Read the model definition and answer for the solid it produces. Units are mm, in the model's axes. Face numbers are marked on the shaded views. A direction names the side the tool comes from. Coordinates: 2 decimals unless noted, no trailing zeros. Write each loop counter-clockwise with the first axis right and the second up, starting at its lowest first coordinate (ties: lowest second). Pieces come first, ordered by that corner, then holes. Notation, with made-up numbers: (29.25, 33) -> (37.25, 33) arc R16 ccw to (37.25, 63) -> close; hole circle Ø10 at (-35, -17). An arc over 180 degrees is marked (long way). Write item = value, one per line. Start each with the question number.
1) Section B-B (z = 3) is taken. Determine the outline of the cut face in (x, y).
2) Find the intervals of material crossed by line 1 along X through (y, z) = (138, 6.75); line 2 along X through (y, z) = (12.5, 5), in increasing order. Write a range as from..to.
3) Section C-C (y = 113.5) is taken. Determine the outline of the cut face in (x, z).
4) Section D-D (y = 40.5) is taken. Determine the outline of the cut face in (x, z), plus the area to 3 significant figures.
5) A tool of negligible diameter and unlimited length cuts with its end or side. For the marked faces 1 and 2, from which of +Z, -Z, +X, -X, +Y, -Y can it reach the whole face along a straight path? Write none if from no direction.
6) Section A-A (x = -9.5) is taken. Determine the outline of the cut face in (y, z), plus the area to 3 significant figures.
7) Flat-ended cylindrical pins translate along their axes: pin 1 Ø1 at (y, z) = (78.5, 4.5) entering from +X; pin 2 Ø3.5 at (y, z) = (-0.5, 4) entering from -X; pin 3 Ø6 at (x, y) = (-15, 128) entering from -Z; pin 4 Ø2 at (y, z) = (-0.5, 2) entering from +X. Find the tip coordinate at first contact, or state that the pin passes through.
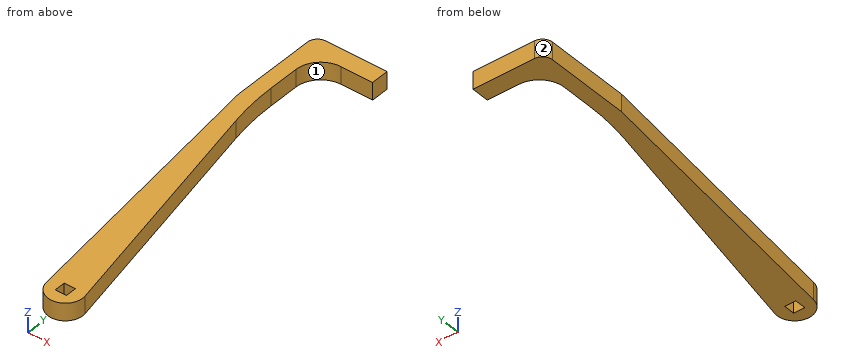
Autodesk Inventor part; units mm, degrees
ref_plane "YZ Plane" through (0, 0, 0) normal (1, 0, 0) x (0, 1, 0)
ref_plane "XZ Plane" through (0, 0, 0) normal (0, 1, 0) x (-1, 0, 0)
ref_plane "XY Plane" through (0, 0, 0) normal (0, 0, 1) x (1, 0, 0)
sketch "Эскиз1" plane through (0, 0, 0) normal (0, 0, 1) x (1, 0, 0)
  circle A0 centre (0.0899, -0.0505) radius 4
  line L0 (-20.8576, 111.2941) -> (-20.8576, 149.3795)
  line L1 (-20.8576, 149.3795) -> (-6.2988, 149.3795)
  line L2 (7.9099, 149.3795) -> (-6.2988, 149.3795)
  line L3 (-14.8576, 142.2545) -> (7.9099, 142.2545)
  line L4 (-14.8576, 142.2545) -> (7.9099, 142.2545)
  line L5 (-14.8576, 109.9334) -> (-14.8576, 142.2545)
  circle A1 centre (0.0899, -0.0505) radius 7
  line L6 (-2.25, -2.25) -> (2.25, -2.25)
  line L7 (2.25, -2.25) -> (2.25, 2.25)
  line L8 (2.25, 2.25) -> (-2.25, 2.25)
  line L9 (-2.25, 2.25) -> (-2.25, -2.25)
  line L10 (-2.25, -2.25) -> (2.25, 2.25) construction
  line L11 (2.25, -2.25) -> (-2.25, 2.25) construction
  line L12 (7.9099, 142.2545) -> (7.9099, 149.3795)
  line L13 (-20.8576, 111.2941) -> (-6.8563, -0.9172)
  line L14 (-14.8576, 109.9334) -> (6.9529, 1.3278)
  point P0 (0, 0)
  dimension "d0" = 14
  dimension "d1" = 4.5
  dimension "d2" = 4.5
extrude "Выдавливание1" add sketch "Эскиз1" along normal blind 7 contours A0 | L0 L1 L2 L12 L3 L5 L14 A1 L13 | A1
fillet "Сопряжение1" radius 10 1 edges at (-14.8576, 142.2545, 3.5)
fillet "Сопряжение2" radius 4 1 edges at (-20.8576, 149.3795, 3.5)
fillet "Сопряжение3" radius 100 1 edges at (-14.8576, 109.9334, 3.5)
properties part number "Arm"
Answer key:
q1.outline = (-20.86, 111.29) -> (-6.86, -0.92) arc R7 ccw (long way) to (6.95, 1.33) -> (-12.9, 100.19) arc R100 cw to (-14.86, 119.88) -> (-14.86, 132.25) arc R10 cw to (-4.86, 142.25) -> (7.91, 142.25) -> (7.91, 149.38) -> (-16.86, 149.38) arc R4 ccw to (-20.86, 145.38) -> close; hole (-2.25, -2.25) -> (2.25, -2.25) -> (2.25, 2.25) -> (-2.25, 2.25) -> close
q2.line_1 = -20.86..-13.04
q2.line_2 = -8.53..4.71
q3.outline = (-20.86, 0) -> (-14.65, 0) -> (-14.65, 7) -> (-20.86, 7) -> close
q4.outline = (-12.02, 0) -> (-0.91, 0) -> (-0.91, 7) -> (-12.02, 7) -> close
q4.area = 77.8 mm^2
q5.face_1 = +Z, -Z, +X
q5.face_2 = +Z, -Z, -X, +Y
q6.outline = (20.27, 0) -> (83.26, 0) -> (83.26, 7) -> (20.27, 7) -> close; (141.11, 0) -> (149.38, 0) -> (149.38, 7) -> (141.11, 7) -> close
q6.area = 499 mm^2
q7.pin_1 = -8.44
q7.pin_2 = -7.13
q7.pin_3 = 0
q7.pin_4 = 7.09
